Build history of the part. All positions in model axes, mm. Face numbers are marked on the shaded views. A direction names the side the tool comes from. Give positions to 0.01 mm unless a question says otherwise; leave off trailing zeros. Order: outer loops, then holes, each group sorted by start corner. A loop starts at its lowest first (then second) coordinate and runs counter-clockwise, first axis right, second up. Notation, with made-up numbers: (19, 29) -> (32, 29) arc R22 ccw to (32, 63) -> close; hole circle Ø10 at (72, 82). An arc over 180 degrees is marked (long way). One line per item, written item: value. Start each with the question number.
(1) Pin check, flat tips, straight feed: pin 1 (4 mm diameter, centred on y = 3.5, z = 20.5, fed in from +X); pin 2 (1.5 mm diameter, centred on x = -24.5, z = 9.5, fed in from -Y); pin 3 (1.5 mm diameter, centred on x = 3.5, y = 3, fed in from -Z). Stop position of each tip, or through.
(2) Saw through at B-B on x = 0. Give the cut face in (y, z), plus the area to 3 significant figures.
(3) Saw through at A-A on z = 0. Give the cut face in (x, y).
(4) Saw through at C-C on y = 4.75. Give the cut face in (x, z), plus the area to 3 significant figures.
(5) Two-plate mould, pull along X, no slides. Class the marked faces 3 and 4: +X half, -X half, draft (parallel to the pull), parting line (faces both ways), or undercut.
(6) Which spindle directions (+Z, -Z, +X, -X, +Y, -Y) get a long thin tool onto all of the face, cutting with end or side? Do the marked faces 1 and 2. Say none if no direction does.
(7) Probe line 1 (X direction, y = 4.5, z = 0.5) (3 decimals); line 2 (X direction, y = 0.45, z = 0); line 3 (Z direction, x = 6, y = 6.25). List the from-to ranges inside material, lowest first.
```python
from build123d import *

# Parameters (mm, degrees)
CROQUIS1_R                 = 32.5
CROQUIS1_R_2               = 25
SALIENTE_EXTRUIR1_DEPTH    = 7
INTERNAL_SEAL_SKETCH_R     = 31
INTERNAL_SEAL_SKETCH_R_2   = 26.5
CORTAR_EXTRUIR1_DEPTH      = 1
INTERNAL_ADJUST_SKETCH_R   = 26.5
INTERNAL_ADJUST_SKETCH_R_2 = 25
CORTAR_EXTRUIR2_DEPTH      = 0.5


with BuildPart() as part:
    # Croquis1 → Saliente-Extruir1 (new body)
    with BuildSketch(Plane(origin=(0, 0, 0), x_dir=(1, 0, 0), z_dir=(0, 1, 0))):
        with Locations(Location((0, 0, 0), (0, 0, 270))):
            Circle(CROQUIS1_R)
        with Locations(Location((0, 0, 0), (0, 0, 270))):
            Circle(CROQUIS1_R_2, mode=Mode.SUBTRACT)
    extrude(amount=SALIENTE_EXTRUIR1_DEPTH)

    # Internal seal sketch → Cortar-Extruir1 (cut)
    with BuildSketch(Plane(origin=(0, 7, 0), x_dir=(1, 0, 0), z_dir=(0, 1, 0))):
        with Locations(Location((0, 0, 0), (0, 0, 270))):
            Circle(INTERNAL_SEAL_SKETCH_R)
        with Locations(Location((0, 0, 0), (0, 0, 270))):
            Circle(INTERNAL_SEAL_SKETCH_R_2, mode=Mode.SUBTRACT)
    cortar_extruir1 = extrude(amount=-CORTAR_EXTRUIR1_DEPTH, mode=Mode.SUBTRACT)

    # Internal adjust sketch → Cortar-Extruir2 (cut)
    with BuildSketch(Plane(origin=(0, 7, 0), x_dir=(1, 0, 0), z_dir=(0, 1, 0))):
        with Locations(Location((0, 0, 0), (0, 0, 270))):
            Circle(INTERNAL_ADJUST_SKETCH_R)
        with Locations(Location((0, 0, 0), (0, 0, 270))):
            Circle(INTERNAL_ADJUST_SKETCH_R_2, mode=Mode.SUBTRACT)
    cortar_extruir2 = extrude(amount=-CORTAR_EXTRUIR2_DEPTH, mode=Mode.SUBTRACT)

    # Simetría1: Cortar-Extruir1, Cortar-Extruir2 across plane
    add(cortar_extruir1.mirror(Plane.ZX.offset(3.5)), mode=Mode.SUBTRACT)
    add(cortar_extruir2.mirror(Plane.ZX.offset(3.5)), mode=Mode.SUBTRACT)


solid = part.part
```
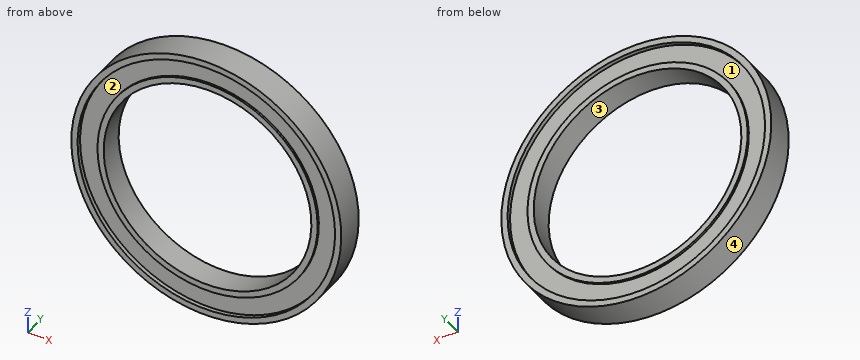
Results below:
1. pin 1: stops at x = 26.72
1. pin 2: stops at y = 0.5
1. pin 3: stops at z = -32.38
2. outline: (0, -32.5) -> (7, -32.5) -> (7, -31) -> (6, -31) -> (6, -26.5) -> (6.5, -26.5) -> (6.5, -25) -> (0.5, -25) -> (0.5, -26.5) -> (1, -26.5) -> (1, -31) -> (0, -31) -> close; (0, 31) -> (1, 31) -> (1, 26.5) -> (0.5, 26.5) -> (0.5, 25) -> (6.5, 25) -> (6.5, 26.5) -> (6, 26.5) -> (6, 31) -> (7, 31) -> (7, 32.5) -> (0, 32.5) -> close
2. area: 84.0 mm²
3. outline: (-32.5, 0) -> (-31, 0) -> (-31, 1) -> (-26.5, 1) -> (-26.5, 0.5) -> (-25, 0.5) -> (-25, 6.5) -> (-26.5, 6.5) -> (-26.5, 6) -> (-31, 6) -> (-31, 7) -> (-32.5, 7) -> close; (25, 0.5) -> (26.5, 0.5) -> (26.5, 1) -> (31, 1) -> (31, 0) -> (32.5, 0) -> (32.5, 7) -> (31, 7) -> (31, 6) -> (26.5, 6) -> (26.5, 6.5) -> (25, 6.5) -> close
4. outline: circle Ø65 at (0, 0); hole circle Ø50 at (0, 0)
4. area: 1,350 mm²
5. face 3: undercut
5. face 4: parting line
6. face 1: +Y
6. face 2: -Y
7. line 1: x = -32.496 to -24.995, 24.995 to 32.496
7. line 2: x = -32.5 to -31, 31 to 32.5
7. line 3: z = -31.94 to -30.41, -25.81 to -24.27, 24.27 to 25.81, 30.41 to 31.94
